```python
from build123d import *

# Parameters (mm, degrees)
F0_R     = 3.5
F1_DEPTH = 4
F2_R     = 4.75
F2_R_2   = 3.5
F3_DEPTH = 1.9
F4_R     = 3.25
F5_DEPTH = 0.8
F6_R     = 0.9
F7_DEPTH = 5.5


with BuildPart() as f1:
    # F0 (on Top) → F1 (new body)
    with BuildSketch(Plane.XY):
        Circle(F0_R)
    extrude(amount=F1_DEPTH)

    # F2 (on face) → F3 (join)
    with BuildSketch(Plane.XY.offset(4)):
        Circle(F2_R)
        Circle(F2_R_2, mode=Mode.SUBTRACT)
        Circle(F2_R_2)
    extrude(amount=F3_DEPTH)

    # F4 (on face) → F5 (join)
    with BuildSketch(Plane.XY.offset(5.9)):
        Circle(F4_R)
    extrude(amount=F5_DEPTH)

    # F6 (on face) → F7 (cut)
    with BuildSketch(Plane(origin=(0, 0, 0), x_dir=(1, 0, 0), z_dir=(0, 0, -1))):
        Circle(F6_R)
    extrude(amount=-F7_DEPTH, mode=Mode.SUBTRACT)


solid = f1.part
```
Input: part model. Units: mm. Frame: model coordinates. A direction names the side the tool comes from. Give positions to 0.01 mm unless a question says otherwise; leave off trailing zeros. Loops run counter-clockwise (first coordinate to the right, second up) from the corner with the lowest first, then second, coordinate; pieces in that order, holes last. Notation, with made-up numbers: M -16,50 L 37,50 A17 cw 37,74 Z; hole C -22,-16.75 d10. An arc over 180 degrees is marked long. Answer as CSV lines item,"result". Start each with the question number.
1. Line query: L1, parallel to Y at x = 0, z = 3.6; L2, parallel to Y at x = 0, z = 4.15; L3, parallel to Z at x = 3, y = -2.25. Output: solid intervals per line, ascending.
2. Section C-C on z = 2.25. Return loops of the section in (x, y), plus the area to 3 significant figures.
3. Section B-B on x = 0. Return loops of the section in (y, z).
4. Reachability of faces 1 (the face through (0.86, -0.27, 2.71)), 2 (the face through (-2.579, -1.978, 6.294)), 3 (the face through (0, 0, 6.7)) from +Z, -Z, +X, -X, +Y, -Y: full face, straight path, thin tool, end or side. Return the list, or none.
5. Section A-A on y = -2.25. Return loops of the section in (x, z).
6. Pin query (flat end, axial travel): P1, Ø1.5, axis at x = 3, z = 1.5, coming from the +Y side; P2, Ø3, axis at y = -2.5, z = 6, coming from the +X side; P3, Ø3, axis at y = 2.5, z = 0.5, coming from the -X side. Return the tip coordinate at first contact, or that it passes through.
7. Pull-direction query (X, two-part tool) for faces 4 (the face through (0, 0, 5.5)), 5 (the face through (2.192, -4.214, 4.937)), 6 (the face through (2, -3, 5.9)); classes: released by +X, released by -X, zero draft, split by the parting line, or undercut.
Computed values:
1,L1,"y = -3.5 to -0.9, 0.9 to 3.5"
1,L2,"y = -4.75 to -0.9, 0.9 to 4.75"
1,L3,"z = 4 to 5.9"
2,outline,"C 0,0 d7; hole C 0,0 d1.8"
2,area,"35.9 mm²"
3,outline,"M -4.75,4 L -3.5,4 L -3.5,0 L -0.9,0 L -0.9,5.5 L 0.9,5.5 L 0.9,0 L 3.5,0 L 3.5,4 L 4.75,4 L 4.75,5.9 L 3.25,5.9 L 3.25,6.7 L -3.25,6.7 L -3.25,5.9 L -4.75,5.9 Z"
4,face 1,"-Z"
4,face 2,"+Z"
4,face 3,"+Z, +X, -X, +Y, -Y"
5,outline,"M -4.18,4 L -2.68,4 L -2.68,0 L 2.68,0 L 2.68,4 L 4.18,4 L 4.18,5.9 L 2.35,5.9 L 2.35,6.7 L -2.35,6.7 L -2.35,5.9 L -4.18,5.9 Z"
6,P1,"stops at y = 2.68"
6,P2,"stops at x = 4.64"
6,P3,"stops at x = -3.35"
7,face 4,"undercut"
7,face 5,"split by the parting line"
7,face 6,"zero draft"
